from build123d import *

# Parameters (mm, degrees)
BOSS_EXTRUDE1_DEPTH = 2
BOSS_EXTRUDE2_DEPTH = 12
BOSS_EXTRUDE3_DEPTH = 3
BOSS_EXTRUDE4_DEPTH = 3
BOSS_EXTRUDE5_START = -2
BOSS_EXTRUDE5_DEPTH = 2
CUT_EXTRUDE1_DEPTH  = 3


with BuildPart() as part:
    # Sketch1 → Boss-Extrude1 (new body)
    with BuildSketch(Plane(origin=(0, 0, 0), x_dir=(1, 0, 0), z_dir=(0, 1, 0))):
        with BuildLine():
            ThreePointArc((0, -3.2), (-3.2, 0), (0, 3.2))
            Line((0, 3.2), (0, 20))
            ThreePointArc((0, 20), (-9.728487163, 17.474453855), (-17, 10.535653753))
            Line((-17, 10.535653753), (-17, -10.535653753))
            ThreePointArc((-17, -10.535653753), (-9.728487163, -17.474453855), (0, -20))
            Line((0, -20), (0, -3.2))
        make_face()
        with BuildLine():
            Line((0, 20), (0, 3.2))
            ThreePointArc((0, 3.2), (2.2627417, 2.2627417), (3.2, 0))
            ThreePointArc((3.2, 0), (2.2627417, -2.2627417), (0, -3.2))
            Line((0, -3.2), (0, -20))
            ThreePointArc((0, -20), (14.142135624, -14.142135624), (20, 0))
            ThreePointArc((20, 0), (14.142135624, 14.142135624), (0, 20))
        make_face()
        with BuildLine():
            Line((-17, -20), (0, -20))
            ThreePointArc((0, -20), (-9.728487163, -17.474453855), (-17, -10.535653753))
            Line((-17, -10.535653753), (-17, -20))
        make_face()
        with BuildLine():
            Line((-20, -20), (-17, -20))
            Line((-17, -20), (-17, -10.535653753))
            ThreePointArc((-17, -10.535653753), (-19.235384062, -5.477225575), (-20, 0))
            Line((-20, 0), (-20, -20))
        make_face()
        with BuildLine():
            Line((-17, -10.535653753), (-17, 10.535653753))
            ThreePointArc((-17, 10.535653753), (-19.235384062, 5.477225575), (-20, 0))
            ThreePointArc((-20, 0), (-19.235384062, -5.477225575), (-17, -10.535653753))
        make_face()
        with BuildLine():
            Line((-17, 10.535653753), (-17, 20))
            Line((-17, 20), (-20, 20))
            Line((-20, 20), (-20, 0))
            ThreePointArc((-20, 0), (-19.235384062, 5.477225575), (-17, 10.535653753))
        make_face()
        with BuildLine():
            ThreePointArc((-17, 10.535653753), (-9.728487163, 17.474453855), (0, 20))
            Line((0, 20), (-17, 20))
            Line((-17, 20), (-17, 10.535653753))
        make_face()
    extrude(amount=BOSS_EXTRUDE1_DEPTH)

    # Sketch1<4> → Boss-Extrude2 (add)
    with BuildSketch(Plane(origin=(0, 0, 0), x_dir=(1, 0, 0), z_dir=(0, 1, 0))):
        with BuildLine():
            Line((-17, 10.535653753), (-17, 20))
            Line((-17, 20), (-20, 20))
            Line((-20, 20), (-20, 0))
            ThreePointArc((-20, 0), (-19.235384062, 5.477225575), (-17, 10.535653753))
        make_face()
        with BuildLine():
            Line((-17, -10.535653753), (-17, 10.535653753))
            ThreePointArc((-17, 10.535653753), (-19.235384062, 5.477225575), (-20, 0))
            ThreePointArc((-20, 0), (-19.235384062, -5.477225575), (-17, -10.535653753))
        make_face()
        with BuildLine():
            Line((-20, -20), (-17, -20))
            Line((-17, -20), (-17, -10.535653753))
            ThreePointArc((-17, -10.535653753), (-19.235384062, -5.477225575), (-20, 0))
            Line((-20, 0), (-20, -20))
        make_face()
    extrude(amount=BOSS_EXTRUDE2_DEPTH)

    # Sketch2 → Boss-Extrude3 (add)
    with BuildSketch(Plane.XY.offset(20)):
        Polygon((-17, 12), (0, 2), (-17, 2), align=None)
    extrude(amount=-BOSS_EXTRUDE3_DEPTH)

    # Sketch3 → Boss-Extrude4 (add)
    with BuildSketch(Plane(origin=(0, 0, -20), x_dir=(-1, 0, 0), z_dir=(0, 0, -1))):
        Polygon((17, 12), (0, 2), (17, 2), align=None)
    extrude(amount=-BOSS_EXTRUDE4_DEPTH)

    # Sketch4 → Boss-Extrude5 (add)
    with BuildSketch(Plane(origin=(0, 2, 0), x_dir=(1, 0, 0), z_dir=(0, 1, 0)).offset(BOSS_EXTRUDE5_START)):
        with BuildLine():
            Line((-2.75, -1.636306817), (-2.75, 0))
            Line((-2.75, 0), (-2.75, 1.636306817))
            ThreePointArc((-2.75, 1.636306817), (-3.2, 0), (-2.75, -1.636306817))
        make_face()
    extrude(amount=BOSS_EXTRUDE5_DEPTH)

    # Sketch5 → Cut-Extrude1 (cut)
    with BuildSketch(Plane(origin=(-17, 0, 0), x_dir=(0, 0, -1), z_dir=(1, 0, 0))):
        with BuildLine():
            ThreePointArc((-10.01, 7), (-8.5, 5.49), (-6.99, 7))
            Line((-6.99, 7), (-10.01, 7))
        make_face()
        with BuildLine():
            Line((-10.01, 7), (-6.99, 7))
            ThreePointArc((-6.99, 7), (-8.5, 8.51), (-10.01, 7))
        make_face()
        with BuildLine():
            ThreePointArc((10.01, 7), (8.5, 8.51), (6.99, 7))
            Line((6.99, 7), (10.01, 7))
        make_face()
        with BuildLine():
            Line((10.01, 7), (6.99, 7))
            ThreePointArc((6.99, 7), (8.5, 5.49), (10.01, 7))
        make_face()
    extrude(amount=-CUT_EXTRUDE1_DEPTH, mode=Mode.SUBTRACT)


solid = part.part
Check sheet for the modelled part. Datum: model origin and axes. Units: mm. A direction names the side the tool comes from. Give positions to 0.01 mm unless a question says otherwise; leave off trailing zeros. Order: outer loops, then holes, each group sorted by start corner. A loop starts at its lowest first (then second) coordinate and runs counter-clockwise, first axis right, second up. Notation, with made-up numbers: M -27,18.25 L 26,18.25 A22 ccw 26,57.25 Z; hole C 89.5,8 d5. An arc over 180 degrees is marked long. Answer as CSV lines item,"result". Start each with the question number.
Item 1: Cross-section at C-C on y = 11. Enter the section's corners in (x, z), plus the area to 3 significant figures.
Item 2: Cross-section at D-D on z = 12. Enter the section's corners in (x, y).
Item 3: Cross-section at B-B on x = -17.5. Enter the section's corners in (y, z).
Item 4: Thickness scan on line 1 (Z direction, x = -8.5, y = 4.75); line 2 (Y direction, x = -18.45, z = 8.5); line 3 (X direction, y = 7.5, z = 6.5). Record the ranges inside material, lowest first. Write a range as [from, to].
Item 5: Gauge pin test, flat ends, axial feed: P1, Ø4, axis at y = 10, z = -14, coming from the +X side; P2, Ø5, axis at x = 0, z = 8, coming from the +Y side; P3, Ø5, axis at y = 3.5, z = 10.5, coming from the +X side. Record the tip position at first contact, or that the pin passes through.
Item 6: Tool access check on faces 4 (the face through (-2.75, 1, 0)), 5 (the face through (-8.62, 7.07, -18.52)), 6 (the face through (-12, 5, -17)). Record the directions out of +Z, -Z, +X, -X, +Y, -Y that give a thin tool (end or side, any length) a straight path to the whole face; none if there is none.
Item 7: Cross-section at A-A on y = 7. Enter the section's corners in (x, z).
Item 8: Mould release check, pull along Z, two halves, no side actions. Record for faces 1 (the face through (-3, 2, 0)), 2 (the face through (-8.62, 7.07, 18.52)), 3 (the face through (-12, 5, 20)): +Z half, -Z half, draft (parallel to the pull), parting line (faces both ways), or undercut.
Established:
1,outline,"M -20,-20 L -15.3,-20 L -15.3,-17 L -17,-17 L -17,17 L -15.3,17 L -15.3,20 L -20,20 Z"
1,area,"130 mm^2"
2,outline,"M -20,0 L 16,0 L 16,2 L -17,2 L -17,12 L -20,12 Z"
3,outline,"M 0,-20 L 12,-20 L 12,20 L 0,20 Z; hole C 7,-8.5 d3.02; hole C 7,8.5 d3.02"
4,line 1,"z = [-20, -17], [17, 20]"
4,line 2,"y = [0, 5.49], [8.51, 12]"
4,line 3,"x = [-20, -17]"
5,P1,"stops at x = -17"
5,P2,"stops at y = 2"
5,P3,"stops at x = 18.1"
6,face 4,"+Y, -Y"
6,face 5,"+Z, -Z, +X, +Y"
6,face 6,"+X, +Y"
7,outline,"M -20,-20 L -8.5,-20 L -8.5,-17 L -17,-17 L -17,-10.01 L -20,-10.01 Z; M -20,-6.99 L -17,-6.99 L -17,6.99 L -20,6.99 Z; M -20,10.01 L -17,10.01 L -17,17 L -8.5,17 L -8.5,20 L -20,20 Z"
8,face 1,"undercut"
8,face 2,"draft"
8,face 3,"+Z half"
